Verification items for the finished model (mm, model axes). A direction names the side the tool comes from. Coordinates: 2 decimals unless noted, no trailing zeros. Loops run counter-clockwise (first coordinate to the right, second up) from the corner with the lowest first, then second, coordinate; pieces in that order, holes last.
Q1. Sectioned sample at A-A (z = -6.5). Enter the section's corners in (x, y).
Q2. Material ranges on probe 1 along Z at (x, y) = (23.5, 22.5); probe 2 along X at (y, z) = (-4, 48.5); probe 3 along Y at (x, z) = (2, 17), recorded low to high.
Q3. Access from +Z, -Z, +X, -X, +Y, -Y to the whole of each face (thin tool, end or side, straight path). Record for faces 1 (the face through (3.442, -5, 31)), 2 (the face through (-2, 44, -21.008)), 3 (the face through (-2, 0, 33)), 4 (the face through (-6.558, -5, 31)).
Q4. Go/stop test with flat-tipped pins: P1, Ø1, axis at x = -33, y = 45.5, coming from the +Z side; P2, Ø8, axis at y = -6, z = 49, coming from the +X side; P3, Ø8, axis at y = -5, z = 55.5, coming from the -X side. Record where each tip stops, or that it passes through.
Q5. Sectioned sample at B-B (y = 6.5). Enter the section's corners in (x, z).
```python
from build123d import *

# Parameters (mm, degrees)
F0_W     = 10
F0_H     = 100
F1_DEPTH = 10
F3_DEPTH = 110


with BuildPart() as f1:
    # F0 (on Front) → F1 (new body)
    with BuildSketch(Plane.XZ):
        with Locations((-1.558005, 31.992308)):
            Rectangle(F0_W, F0_H)
    extrude(amount=F1_DEPTH)

    # F2 (on face) → F3 (join)
    with BuildSketch(Plane.XZ.offset(10)):
        Polygon((3.441995, -18.007692), (-6.558005, -18.007692), (-61.558005, -18.007692), (-61.558005, -21.007692), (58.441995, -21.007692), (58.441995, -18.007692), align=None)
    extrude(amount=-F3_DEPTH)


solid = f1.part
```
Geometry check:
1. outline: (-6.56, -10) - (3.44, -10) - (3.44, 0) - (-6.56, 0) - close
2. probe 1: z = -21.01 to -18.01
2. probe 2: x = -6.56 to 3.44
2. probe 3: y = -10 to 0
3. face 1: +Z, +X, +Y, -Y
3. face 2: -Z, +X, -X, +Y, -Y
3. face 3: +Z, +X, -X, +Y
3. face 4: +Z, -X, +Y, -Y
4. P1: stops at z = -18.01
4. P2: stops at x = 3.44
4. P3: stops at x = -6.56
5. outline: (-61.56, -21.01) - (58.44, -21.01) - (58.44, -18.01) - (-61.56, -18.01) - close
